Answer from the drawing. Dimensions are ordinates in mm from the lowest x, y and z of the part. A direction names the side the tool comes from. Give positions to 0.01 mm unless a question says otherwise; leave off trailing zeros. Write each loop counter-clockwise with the first axis right and the second up, starting at its lowest first coordinate (ties: lowest second). Pieces come first, ordered by that corner, then holes. Notation, with made-up numbers: (68, -34) - (105, -34) arc R20 cw to (105, -6) - close; hole circle Ø7 at (-29.5, 51.5). An arc over 180 degrees is marked (long way). Answer as a JSON object with one key per item and string values. Group by question number.
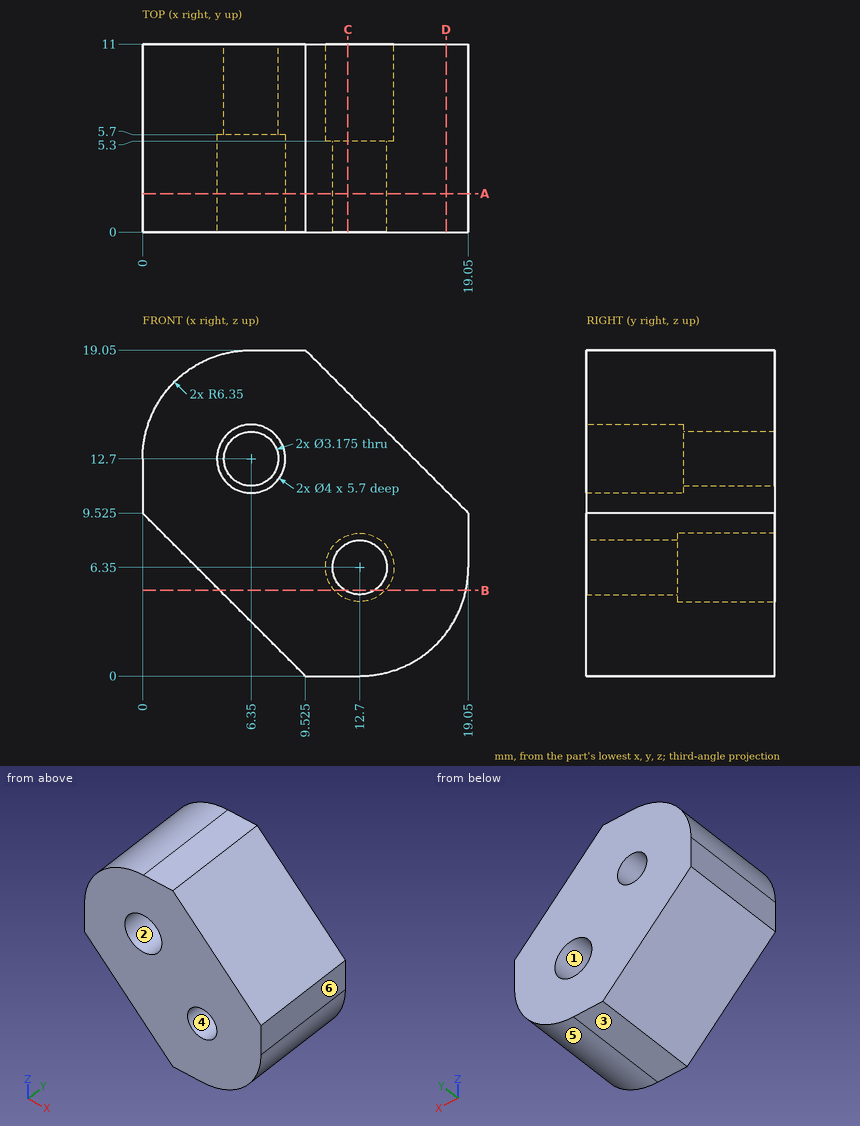
1) Find section D-D, the plane x = 17.75. Write down the section's boundary in (y, z) (3 decimals), and give its area (3 significant figures).
2) Find section A-A, the plane y = 2.25. Give the number of separate pieces and of enclosed holes in the cut face, and give its area (3 significant figures).
3) Which of the six approach directions +Z, -Z, +X, -X, +Y, -Y give full straight-line access (tool end or side, diameter ignored) to the marked faces 1, 2 and 3?
4) Find section C-C, the plane x = 12. Write down the section's boundary in (y, z) (1 decimal).
5) Find section B-B, the plane z = 5. Write down the section's boundary in (x, y) (3 decimals).
6) For a pull along Z with two mould halves and no side action, classify the marked faces 4, 5 and 6 as released by +Z, released by -Z, zero draft, split by the parting line, or undercut.
7) Flat-ended cylindrical pins translate along their axes: pin 1 Ø2.5 at (x, z) = (6.35, 12.7) entering from -Y; pin 2 Ø3 at (x, z) = (12.5, 6) entering from +Y; pin 3 Ø3 at (y, z) = (8.5, 13) entering from +X (3 decimals). Find the tip coordinate at first contact, or state that the pin passes through.
8) Find the intervals of material crossed by line 1 (Y direction, x = 8, z = 13); line 2 (X direction, y = 6.5, z = 5) (3 decimals); line 3 (Z direction, x = 7.25, y = 1.5) (3 decimals), in increasing order. Write a range as [from, to].
Values follow:
{
 "1": {"outline": "(0, 2.5) - (11, 2.5) - (11, 10.825) - (0, 10.825) - close", "area": "91.6 mm2"},
 "2": {"separate pieces": "1", "enclosed holes": "2", "area": "234 mm2"},
 "3": {"face 1": "+Y", "face 2": "-Y", "face 3": "-Z, +X, -X, +Y, -Y"},
 "4": {"outline": "(0, 0) - (11, 0) - (11, 4.5) - (5.3, 4.5) - (5.3, 4.9) - (0, 4.9) - close; (0, 7.8) - (5.3, 7.8) - (5.3, 8.2) - (11, 8.2) - (11, 16.6) - (0, 16.6) - close"},
 "5": {"outline": "(4.525, 0) - (11.865, 0) - (11.865, 5.3) - (11.224, 5.3) - (11.224, 11) - (4.525, 11) - close; (13.535, 0) - (18.905, 0) - (18.905, 11) - (14.176, 11) - (14.176, 5.3) - (13.535, 5.3) - close"},
 "6": {"face 4": "undercut", "face 5": "released by -Z", "face 6": "zero draft"},
 "7": {"pin 1": "passes through", "pin 2": "stops at y = 5.3", "pin 3": "stops at x = 17.075"},
 "8": {"line 1": "y = [5.7, 11]", "line 2": "x = [4.525, 11.224], [14.176, 18.905]", "line 3": "z = [2.275, 10.914], [14.486, 19.05]"}
}
